from build123d import *

# Parameters (mm, degrees)
SKETCH1_W                      = 100
SKETCH1_H                      = 100
BOSS_EXTRUDE3_DEPTH            = 6.35
M3_CLEARANCE_HOLE1_D           = 3.4
M3_CLEARANCE_HOLE1_CSINK_D     = 3.45
M3_CLEARANCE_HOLE1_CSINK_ANGLE = 90


with BuildPart() as part:
    # Sketch1 → Boss-Extrude3 (new body)
    with BuildSketch(Plane(origin=(0, 0, 0), x_dir=(1, 0, 0), z_dir=(0, 1, 0))):
        Rectangle(SKETCH1_W, SKETCH1_H)
    extrude(amount=BOSS_EXTRUDE3_DEPTH)

    # M3 Clearance Hole1 (through all)
    with Locations(Plane(origin=(0, 6.35, 0), x_dir=(1, 0, 0), z_dir=(0, 1, 0))):
        with Locations((-46.825, 35), (-35, 46.825), (35, 46.825), (46.825, 35), (46.825, -35), (35, -46.825), (-35, -46.825), (-46.825, -35)):
            CounterSinkHole(M3_CLEARANCE_HOLE1_D / 2, M3_CLEARANCE_HOLE1_CSINK_D / 2, counter_sink_angle=M3_CLEARANCE_HOLE1_CSINK_ANGLE)


solid = part.part
Could you check a few things on this model? Use its own coordinates, in mm. Give positions to 0.01 mm unless a question says otherwise; leave off trailing zeros. Loops run counter-clockwise (first coordinate to the right, second up) from the corner with the lowest first, then second, coordinate; pieces in that order, holes last. Notation, with made-up numbers: (19.25, -23) -> (29.25, -23) arc R27 ccw to (29.25, 6) -> close; hole circle Ø9 at (21, 32.25). An arc over 180 degrees is marked (long way). Answer as CSV lines item,"result". Start each with the question number.
(1) I need wall thicknesses on probe 1 along X at (y, z) = (5.25, -35) (3 decimals). Which ranges of the line are inside material? Lowest first, please.
(2) If we section it at B-B on z = 35: Write out the boundary of the cut face in (x, y) (3 decimals), then the cut area to 3 significant figures.
(3) If we section it at A-A on x = -35: Write out the boundary of the cut face in (y, z) (3 decimals).
(4) We'd pull the mould along Z, two halves only. Please class faces 1 (the flat face through (-1, 3, -50)), 2 (the flat face through (50, 3, 1)), 3 (the cylindrical face through (45.255, 3.118, -34.349)): released by +Z, released by -Z, zero draft, split by the parting line, or undercut.
Computed:
1,probe 1,"x = -50 to -48.525, -45.125 to 45.125, 48.525 to 50"
2,outline,"(-50, 0) -> (-48.525, 0) -> (-48.525, 6.325) -> (-48.55, 6.35) -> (-50, 6.35) -> close; (-45.125, 0) -> (45.125, 0) -> (45.125, 6.325) -> (45.1, 6.35) -> (-45.1, 6.35) -> (-45.125, 6.325) -> close; (48.525, 0) -> (50, 0) -> (50, 6.35) -> (48.55, 6.35) -> (48.525, 6.325) -> close"
2,area,"592 mm2"
3,outline,"(0, -50) -> (6.35, -50) -> (6.35, -48.55) -> (6.325, -48.525) -> (0, -48.525) -> close; (0, -45.125) -> (6.325, -45.125) -> (6.35, -45.1) -> (6.35, 45.1) -> (6.325, 45.125) -> (0, 45.125) -> close; (0, 48.525) -> (6.325, 48.525) -> (6.35, 48.55) -> (6.35, 50) -> (0, 50) -> close"
4,face 1,"released by -Z"
4,face 2,"zero draft"
4,face 3,"undercut"
